from build123d import *

# Parameters (mm, degrees)
F0_W      = 304.8
F0_H      = 101.6
F1_DEPTH  = 6.35
F2_R      = 14.2875
F3_DEPTH  = 6.35
F5_R      = 2.413
F6_DEPTH  = 6.35
F7_R      = 3.1115
F8_DEPTH  = 6.35
F9_R      = 3.1115
F10_DEPTH = 6.35
F11_R     = 3.1115
F12_DEPTH = 6.35
F13_R     = 3.1115
F14_DEPTH = 6.35
F15_R     = 14.2875
F16_DEPTH = 6.35
F17_R     = 3.1115
F19_DEPTH = 6.35
F18_R     = 3.1115
F20_DEPTH = 6.35
F21_SIZE  = 50.8
F23_DEPTH = 6.35


with BuildPart() as f1:
    # F0 (on Top) → F1 (new body)
    with BuildSketch(Plane.XY):
        with Locations((79.710026, -8.171286)):
            Rectangle(F0_W, F0_H)
    extrude(amount=F1_DEPTH)

    # F2 (on face) → F3 (cut)
    with BuildSketch(Plane.XY.offset(6.35)):
        with Locations((54.310026, -8.171286)):
            Circle(F2_R)
    extrude(amount=-F3_DEPTH, mode=Mode.SUBTRACT)

    # F5 (on face) → F6 (cut)
    with BuildSketch(Plane.XY.offset(6.35)):
        with Locations((36.580826, -25.900486)):
            Circle(F5_R)
        with Locations((72.039226, 9.557914)):
            Circle(F5_R)
    extrude(amount=-F6_DEPTH, mode=Mode.SUBTRACT)

    # F7 (on face) → F8 (cut)
    with BuildSketch(Plane.XY):
        with Locations((27.322526, 29.928714)):
            Circle(F7_R)
    extrude(amount=F8_DEPTH, mode=Mode.SUBTRACT)

    # F9 (on face) → F10 (cut)
    with BuildSketch(Plane.XY.offset(6.35)):
        with Locations((219.410026, 29.928714)):
            Circle(F9_R)
    extrude(amount=-F10_DEPTH, mode=Mode.SUBTRACT)

    # F11 (on face) → F12 (cut)
    with BuildSketch(Plane.XY.offset(6.35)):
        with Locations((27.330443, -46.271286)):
            Circle(F11_R)
    extrude(amount=-F12_DEPTH, mode=Mode.SUBTRACT)

    # F13 (on face) → F14 (cut)
    with BuildSketch(Plane.XY.offset(6.35)):
        with Locations((219.410026, -46.271286)):
            Circle(F13_R)
    extrude(amount=-F14_DEPTH, mode=Mode.SUBTRACT)

    # F15 (on face) → F16 (cut)
    with BuildSketch(Plane.XY.offset(6.35)):
        with Locations((181.310026, -8.171286)):
            Circle(F15_R)
    extrude(amount=-F16_DEPTH, mode=Mode.SUBTRACT)

    # F17 (on Top) → F19 (cut)
    with BuildSketch(Plane.XY):
        with Locations((92.410026, 17.863714)):
            Circle(F17_R)
    extrude(amount=F19_DEPTH, mode=Mode.SUBTRACT)

    # F18 (on Top) → F20 (cut)
    with BuildSketch(Plane.XY):
        with Locations((92.410026, -34.206286)):
            Circle(F18_R)
    extrude(amount=F20_DEPTH, mode=Mode.SUBTRACT)

    # F21
    f21_edges = [f1.edges().sort_by_distance(p)[0] for p in [
        (-72.689974, 42.628714, 3.175),
    ]]
    chamfer(f21_edges, length=F21_SIZE)

    # F22 (on face) → F23 (cut)
    with BuildSketch(Plane(origin=(0, 0, 0), x_dir=(1, 0, 0), z_dir=(0, 0, -1))):
        with BuildLine():
            ThreePointArc((-40.971884, 15.549221), (-47.080201, 16.76424), (-41.90182, 13.304157))
            ThreePointArc((-41.90182, 13.304157), (-41.213566, 14.334201), (-40.971884, 15.549221))
        make_face()
        with BuildLine():
            ThreePointArc((-33.819589, 5.221926), (-35.679461, 0.731798), (-33.819589, -3.75833))
            Line((-33.819589, -3.75833), (-29.329461, 0.731798))
            Line((-29.329461, 0.731798), (-33.819589, 5.221926))
        make_face()
        with BuildLine():
            Line((-33.819589, 5.221926), (-29.329461, 0.731798))
            Line((-29.329461, 0.731798), (-24.839333, 5.221926))
            ThreePointArc((-24.839333, 5.221926), (-29.329461, 7.081798), (-33.819589, 5.221926))
        make_face()
        with BuildLine():
            Line((-24.839333, 5.221926), (-29.329461, 0.731798))
            Line((-29.329461, 0.731798), (-24.839333, -3.75833))
            ThreePointArc((-24.839333, -3.75833), (-23.462826, -1.698242), (-22.979461, 0.731798))
            ThreePointArc((-22.979461, 0.731798), (-23.462826, 3.161838), (-24.839333, 5.221926))
        make_face()
        with BuildLine():
            Line((-29.329461, 0.731798), (-33.819589, -3.75833))
            ThreePointArc((-33.819589, -3.75833), (-29.329461, -5.618202), (-24.839333, -3.75833))
            Line((-24.839333, -3.75833), (-29.329461, 0.731798))
        make_face()
        with BuildLine():
            ThreePointArc((-11.337039, -14.085625), (-13.297019, -11.152307), (-16.757103, -11.840561))
            ThreePointArc((-16.757103, -11.840561), (-15.727059, -17.018942), (-11.337039, -14.085625))
        make_face()
    extrude(amount=-F23_DEPTH, mode=Mode.SUBTRACT)


solid = f1.part
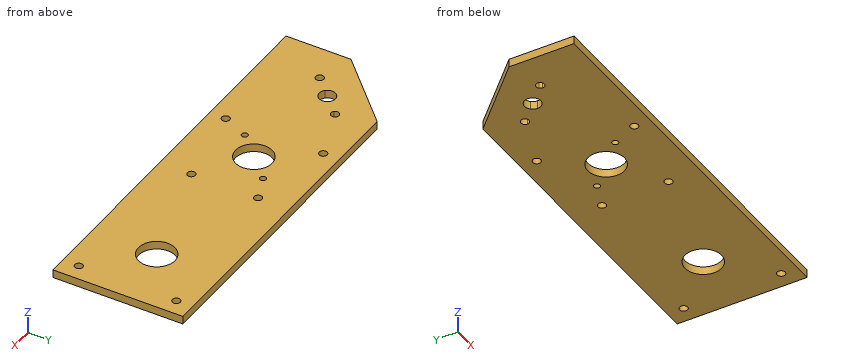
Work out the finished part from the listing and answer in its coordinate system (mm). Round coordinates to 2 decimals unless told otherwise and drop trailing zeros. Loops run counter-clockwise (first coordinate to the right, second up) from the corner with the lowest first, then second, coordinate; pieces in that order, holes last. Notation, with made-up numbers: M -21.5,-16.75 L -0.5,-16.75 A36 ccw -0.5,18.25 Z; hole C -16,-19.5 d10. An arc over 180 degrees is marked long. One line per question, with ' | ' between items. Start each with the question number.
(1) Flat-ended cylindrical pins translate along their axes: pin 1 Ø1.5 at (x, y) = (0.5, 9) entering from -Z; pin 2 Ø3.5 at (x, y) = (92.41, -34.21) entering from +Z (3 decimals). Find the tip coordinate at first contact, or state that the pin passes through.
(2) A cutting plane is placed at A-A on x = 51. Write down the section's boundary in (y, z).
(3) Find the intervals of material crossed by line 1 (Y direction, x = 181.5, z = 2.25); line 2 (X direction, y = -17, z = 2); line 3 (X direction, y = 15, z = 3), in increasing order.
(4) A cutting plane is placed at B-B on z = 4. Give the number of separate pieces and of enclosed holes in the cut face, plus the area to 3 significant figures.
Geometry check:
1) pin 1: stops at z = 0 | pin 2: passes through
2) outline: M -58.97,0 L -22.07,0 L -22.07,6.35 L -58.97,6.35 Z; M 5.73,0 L 42.63,0 L 42.63,6.35 L 5.73,6.35 Z
3) line 1: y = -58.97 to -22.46, 6.11 to 42.63 | line 2: x = -72.69 to -46.97, -41.32 to 43.08, 65.54 to 170.08, 192.54 to 232.11 | line 3: x = -49.52 to -17.55, -11.47 to 91.19, 93.63 to 232.11
4) separate pieces: 1 | enclosed holes: 13 | area: 28,000 mm²
